from build123d import *

# Parameters (mm, degrees)
EXT_PEDAL_STEM_DEPTH     = 20.955
EXT_FOOT_SIDE_DEPTH      = 26.67
CUT_FOOT_PLAN_DEPTH      = 126.067228803
CUT_FOOT_PLAN_DEPTH_BACK = 126.067228803
SK_RIBS_STEM_R           = 0.635
EXT_RIBS_STEM_DEPTH      = 17.145
SK_RIBS_FOOT_R           = 0.635
EXT_RIBS_FOOT_DEPTH      = 22.225


with BuildPart() as part:
    # Sk_pedal_stem → Ext_pedal_stem (new, symmetric)
    with BuildSketch(Plane.XY):
        with BuildLine():
            Line((62.5221, 30.214062), (62.5221, 54.861968))
            ThreePointArc((62.5221, 54.861968), (77.145265739, 50.212536002), (91.40698, 44.550584))
            ThreePointArc((91.40698, 44.550584), (91.550950572, 44.483878693), (91.691968, 44.411138))
            ThreePointArc((91.691968, 44.411138), (92.690956134, 43.975699122), (93.6879, 43.5356))
            Line((93.6879, 43.5356), (93.6879, 36.191698))
            ThreePointArc((93.6879, 36.191698), (92.609350592, 33.535520735), (89.984326, 32.383222))
            Line((89.984326, 32.383222), (69.311266, 31.805626))
            ThreePointArc((69.311266, 31.805626), (65.835901534, 31.354435095), (62.5221, 30.214062))
        make_face()
    extrude(amount=EXT_PEDAL_STEM_DEPTH, both=True)

    # Sk_foot_side → Ext_foot_side (add, symmetric)
    with BuildSketch(Plane.XY):
        with BuildLine():
            Line((93.6879, 35.071812), (93.6879, 42.118788))
            ThreePointArc((93.6879, 42.118788), (94.090678285, 43.046595361), (95.043498, 43.385994))
            ThreePointArc((95.043498, 43.385994), (99.464687923, 43.686511406), (103.64216, 45.16501))
            ThreePointArc((103.64216, 45.16501), (107.36259935, 45.018864691), (109.1819, 41.7703))
            Line((109.1819, 41.7703), (109.1819, 35.4203))
            ThreePointArc((109.1819, 35.4203), (107.362602336, 32.171730436), (103.64216, 32.02559))
            ThreePointArc((103.64216, 32.02559), (99.464578688, 33.503560617), (95.043498, 33.804606))
            ThreePointArc((95.043498, 33.804606), (94.090614283, 34.143936173), (93.6879, 35.071812))
        make_face()
    extrude(amount=EXT_FOOT_SIDE_DEPTH, both=True)

    # Sk_foot_plan_trim → Cut_foot_plan (cut, two sides: drawn at the far end of the back side and taken through both)
    with BuildSketch(Plane(origin=(0, 0, 0), x_dir=(1, 0, 0), z_dir=(0, 1, 0)).offset(-CUT_FOOT_PLAN_DEPTH_BACK)):
        with BuildLine():
            Line((94.7039, -26.67), (96.87306, -26.67))
            ThreePointArc((96.87306, -26.67), (98.633684187, -26.421041098), (100.25634, -25.693878))
            ThreePointArc((100.25634, -25.693878), (104.672679306, -22.171677589), (108.200952, -17.760188))
            ThreePointArc((108.200952, -17.760188), (108.932068295, -16.134088594), (109.1819, -14.36878))
            Line((109.1819, -14.36878), (109.1819, 14.36878))
            ThreePointArc((109.1819, 14.36878), (108.931624488, 16.133960225), (108.200952, 17.760188))
            ThreePointArc((108.200952, 17.760188), (104.672363352, 22.1713612), (100.25634, 25.693878))
            ThreePointArc((100.25634, 25.693878), (98.633741991, 26.421241452), (96.87306, 26.67))
            Line((96.87306, 26.67), (94.7039, 26.67))
            ThreePointArc((94.7039, 26.67), (93.98547951, 26.37242049), (93.6879, 25.654))
            Line((93.6879, 25.654), (93.6879, 40.64))
            Line((93.6879, 40.64), (119.38, 40.64))
            Line((119.38, 40.64), (119.38, -40.64))
            Line((119.38, -40.64), (93.6879, -40.64))
            Line((93.6879, -40.64), (93.6879, -25.654))
            ThreePointArc((93.6879, -25.654), (93.98547951, -26.37242049), (94.7039, -26.67))
        make_face()
    extrude(amount=CUT_FOOT_PLAN_DEPTH + CUT_FOOT_PLAN_DEPTH_BACK, mode=Mode.SUBTRACT)

    # Sk_ribs_stem → Ext_ribs_stem (add, symmetric)
    with BuildSketch(Plane.XY):
        with Locations((65.6971, 53.61178)):
            Circle(SK_RIBS_STEM_R)
        with Locations((68.8721, 52.53228)):
            Circle(SK_RIBS_STEM_R)
        with Locations((72.0471, 51.64836)):
            Circle(SK_RIBS_STEM_R)
    extrude(amount=EXT_RIBS_STEM_DEPTH, both=True)

    # Sk_ribs_foot → Ext_ribs_foot (add, symmetric)
    with BuildSketch(Plane.XY):
        with Locations((96.2279, 43.2943)):
            Circle(SK_RIBS_FOOT_R)
        with Locations((98.7679, 43.5356)):
            Circle(SK_RIBS_FOOT_R)
        with Locations((101.3079, 44.13504)):
            Circle(SK_RIBS_FOOT_R)
    extrude(amount=EXT_RIBS_FOOT_DEPTH, both=True)


solid = part.part
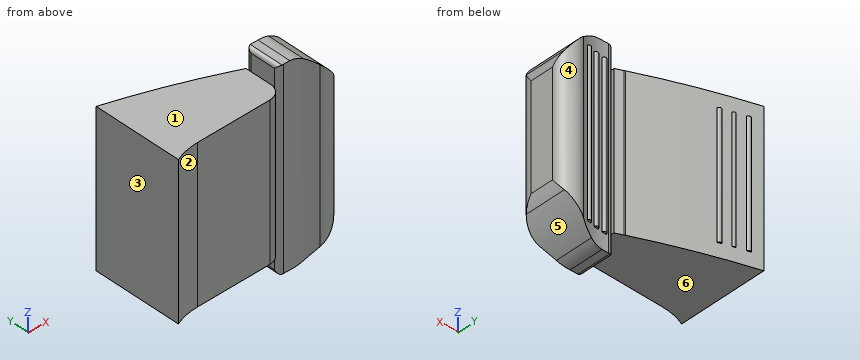
Can you work these out from the model? Positions are in its coordinate system, mm. Face numbers are marked on the shaded views. A direction names the side the tool comes from. Coordinates: 2 decimals unless noted, no trailing zeros. Loops run counter-clockwise (first coordinate to the right, second up) from the corner with the lowest first, then second, coordinate; pieces in that order, holes last. Notation, with made-up numbers: (39.5, 73.5) - (93.5, 73.5) arc R23 cw to (93.5, 107.5) - close; hole circle Ø1 at (-19.75, 7.25). An arc over 180 degrees is marked (long way). Put each result on its own line as item: value. Start each with the question number.
Item 1: If I drill on line 1 along Z through (x, y) = (90, 34.75) (3 decimals); line 2 along X through (y, z) = (37.75, -15); line 3 along Y through (x, z) = (100, -1.5), over which ranges is the centre line in solid material (lowest first)?
Item 2: If we mould it in two halves opening along X, with no side actions, what happens to the marked faces 4, 5 and 6? For each: +X half, -X half, draft (parallel to the pull), parting line (faces both ways), or undercut.
Item 3: For pin 1 (6 mm diameter, centred on x = 104.5, z = -2, fed in from -Y); pin 2 (0.5 mm diameter, centred on x = 65.5, y = 54, fed in from +Z) (3 decimals); pin 3 (0.6 mm diameter, centred on x = 72, y = 52, fed in from -Z) (3 decimals), each with a flat end and sliding along its axis, tell me the tip position at first contact or that it passes through.
Item 4: Suppose I cut it at A-A (y = 39.5). Please give me the cut outline in (x, z) (3 decimals), and give its area (3 significant figures).
Item 5: Suppose I cut it at C-C (x = 87). Please give me the cut outline in (y, z) (3 decimals).
Item 6: Which directions (+Z, -Z, +X, -X, +Y, -Y) give clear straight access to the entire face, cutting with the end or side of a thin tool? Please do the marked faces 1, 2 and 3.
Here are the results:
1. line 1: -20.955 to 20.955
1. line 2: 62.52 to 109.15
1. line 3: 33.38 to 43.81
2. face 4: undercut
2. face 5: +X half
2. face 6: draft
3. pin 1: y = 31.61
3. pin 2: z = 20.955
3. pin 3: z = -20.955
4. outline: (62.522, -20.955) - (93.688, -20.955) - (93.688, -25.654) arc R1.016 ccw to (94.704, -26.67) - (96.873, -26.67) arc R6.348 ccw to (100.256, -25.694) arc R25.408 ccw to (108.201, -17.76) arc R6.356 ccw to (109.182, -14.369) - (109.182, 14.374) arc R6.345 ccw to (108.201, 17.76) arc R25.39 ccw to (100.256, 25.694) arc R6.353 ccw to (96.873, 26.67) - (94.704, 26.67) arc R1.016 ccw to (93.688, 25.654) - (93.688, 20.955) - (62.522, 20.955) - close
4. area: 2,040 mm²
5. outline: (32.3, -20.955) - (46.424, -20.955) - (46.424, 20.955) - (32.3, 20.955) - close
6. face 1: +Z, -X, +Y, -Y
6. face 2: +Z, -Z, -Y
6. face 3: +Z, -Z, -X, +Y, -Y
